Check sheet for the drawn part. Datum: minimum x, y, z corner. Units: mm. A direction names the side the tool comes from. Round coordinates to 2 decimals unless told otherwise and drop trailing zeros. Write each loop counter-clockwise with the first axis right and the second up, starting at its lowest first coordinate (ties: lowest second). Pieces come first, ordered by that corner, then holes. Notation, with made-up numbers: (87.25, 10.25) - (125.25, 10.25) arc R18 cw to (125.25, 41.25) - close; hole circle Ø11 at (71.5, -16.75). An arc over 180 degrees is marked (long way). Answer as a JSON object with one key per item and string values.
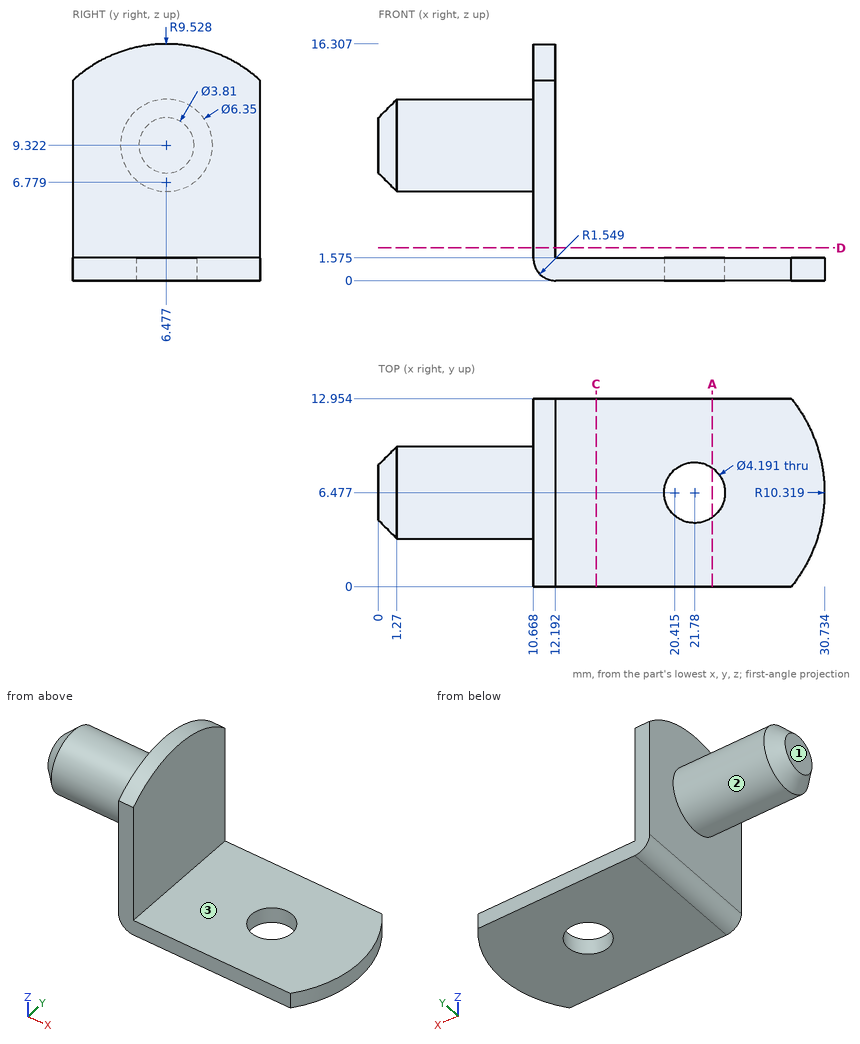
Q1. Section check D-D, the plane z = 2.25. Record the cut outline in (x, y) (1 decimal).
Geometry check:
{"outline": "(10.7, 0) - (12.2, 0) - (12.2, 13) - (10.7, 13) - close"}
Q2. Section check A-A, the plane x = 23. Record the cut outline in (y, z) (1 decimal).
Geometry check:
{"outline": "(0, 0) - (4.8, 0) - (4.8, 1.6) - (0, 1.6) - close; (8.2, 0) - (13, 0) - (13, 1.6) - (8.2, 1.6) - close"}
Q3. Material ranges on line 1 along X through (y, z) = (10, 11); line 2 along Z through (x, y) = (20, 10.25) (1 decimal); line 3 along Z through (x, y) = (6, 6.25) (1 decimal), recorded low to high. Write a range as [from, to].
Geometry check:
{"line 1": "x = [10.67, 12.19]", "line 2": "z = [0, 1.6]", "line 3": "z = [6.2, 12.5]"}
Q4. Set-up check for the marked faces 1, 2 and 3: record each of +Z, -Z, +X, -X, +Y, -Y from which the full face is reachable in a straight line by a thin tool's end or side.
Geometry check:
{"face 1": "+Z, -Z, -X, +Y, -Y", "face 2": "-X", "face 3": "+Z, +X, +Y, -Y"}
Q5. Section check C-C, the plane x = 15. Record the cut outline in (y, z) (1 decimal), then the cut area to 3 significant figures.
Geometry check:
{"outline": "(0, 0) - (13, 0) - (13, 1.6) - (0, 1.6) - close", "area": "20.4 mm2"}
Q6. Gauge pin test, flat ends, axial feed: P1, Ø5, axis at y = 9, z = 7, coming from the +X side; P2, Ø1.5, axis at x = 15, y = 10, coming from the -Z side; P3, Ø5, axis at x = 5, y = 5, coming from the -Z side; P4, Ø4, axis at y = 10.5, z = 13.5, coming from the -X side. Record the tip position at first contact, or that the pin passes through.
Geometry check:
{"P1": "stops at x = 12.19", "P2": "stops at z = 0", "P3": "stops at z = 6.15", "P4": "stops at x = 10.67"}
